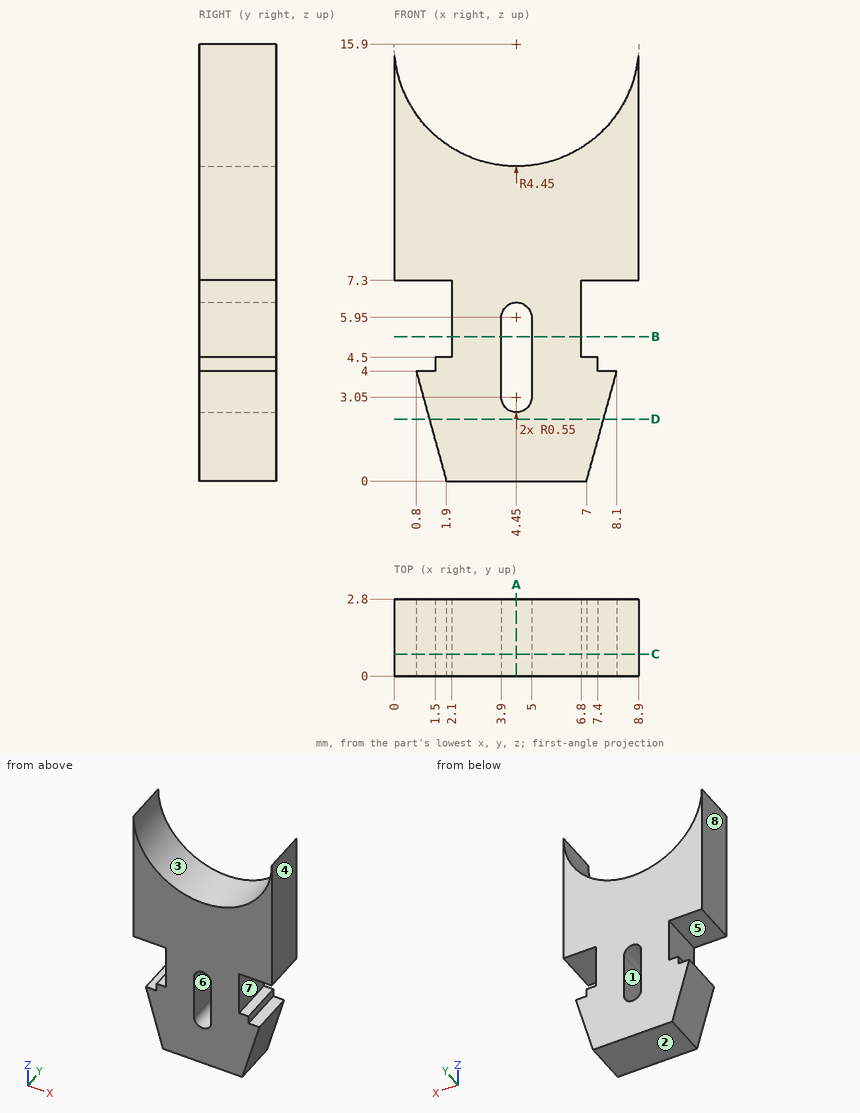
The figure shows three views and two pictorial views of one solid part (mm, origin at its lowest corner). Answer the questions. A direction names the side the tool comes from. Coordinates: 2 decimals unless noted, no trailing zeros. Write each loop counter-clockwise with the first axis right and the second up, starting at its lowest first coordinate (ties: lowest second). Pieces come first, ordered by that corner, then holes.
1. For the marked faces 4, 5, 6, 7 and 8, determine the directions among +Z, -Z, +X, -X, +Y, -Y from which every point of the face is accessible in a straight line to the end or side of a thin tool.
Results list:
face 4: +Z, -Z, +X, +Y, -Y
face 5: -X, +Y, -Y
face 6: +Y, -Y
face 7: +X, +Y, -Y
face 8: +Z, -Z, -X, +Y, -Y
2. The part is cut by section C-C, the plane y = 0.8. Write down the section's boundary in (x, z), and give its area (3 significant figures).
Results list:
outline: (0, 7.3) - (2.1, 7.3) - (2.1, 4.5) - (1.5, 4.5) - (1.5, 4) - (0.8, 4) - (1.9, 0) - (7, 0) - (8.1, 4) - (7.4, 4) - (7.4, 4.5) - (6.8, 4.5) - (6.8, 7.3) - (8.9, 7.3) - (8.9, 15.9) arc R4.45 cw to (0, 15.9) - close; hole (3.9, 3.05) arc R0.55 ccw to (5, 3.05) - (5, 5.95) arc R0.55 ccw to (3.9, 5.95) - close
area: 82.2 mm2
3. Flat-ended cylindrical pins translate along their axes: pin 1 (0.6 mm diameter, centred on y = 2, z = 4.5, fed in from -X); pin 2 (1.5 mm diameter, centred on x = 7, y = 2, fed in from +Z); pin 3 (0.7 mm diameter, centred on x = 2, y = 1.5, fed in from +Z). Find the tip coordinate at first contact, or state that the pin passes through.
Results list:
pin 1: stops at x = 1.5
pin 2: stops at z = 12.91
pin 3: stops at z = 12.44
4. Consider line 1 along X through (y, z) = (0.3, 5.5); line 2 along X through (y, z) = (1.4, 4.25); line 3 along Z through (x, y) = (2, 0.75). Determine where each line is inside the solid, lowest interval first.
Results list:
line 1: x = 2.1 to 3.9, 5 to 6.8
line 2: x = 1.5 to 3.9, 5 to 7.4
line 3: z = 0 to 4.5, 7.3 to 12.19
5. For a pull along Z with two mould halves and no side action, classify the marked faces 1, 2 and 3 as +Z half, -Z half, draft (parallel to the pull), parting line (faces both ways), or undercut.
Results list:
face 1: undercut
face 2: -Z half
face 3: +Z half
6. The part is cut by section D-D, the plane z = 2.25. Write down the section's boundary in (x, y).
Results list:
outline: (1.28, 0) - (7.62, 0) - (7.62, 2.8) - (1.28, 2.8) - close
7. The part is cut by section B-B, the plane z = 5.25. Write down the section's boundary in (x, y), and give its area (3 significant figures).
Results list:
outline: (2.1, 0) - (3.9, 0) - (3.9, 2.8) - (2.1, 2.8) - close; (5, 0) - (6.8, 0) - (6.8, 2.8) - (5, 2.8) - close
area: 10.1 mm2
8. The part is cut by section A-A, the plane x = 4.45. Write down the section's boundary in (y, z).
Results list:
outline: (0, 0) - (2.8, 0) - (2.8, 2.5) - (0, 2.5) - close; (0, 6.5) - (2.8, 6.5) - (2.8, 11.45) - (0, 11.45) - close
